from build123d import *

# Parameters (mm, degrees)
F0_W      = 482.6
F0_H      = 482.6
F1_DEPTH  = 12.8524
F2_W      = 330.2
F2_H      = 12.8524
F2_W_2    = 76.2
F3_DEPTH  = 50.8
F4_W      = 330.2
F4_H      = 12.8524
F4_W_2    = 76.2
F5_DEPTH  = 50.8
F8_W      = 127
F8_H      = 74.6771698952
F8_H_2    = 75.1828301048
F9_W      = 127
F9_H      = 74.6771698952
F10_DEPTH = 25.4
F12_DEPTH = 50.8
F13_DEPTH = 50.8
F14_R     = 30.353
F15_DEPTH = 25.4


with BuildPart() as f1:
    # F0 (on Top) → F1 (new body)
    with BuildSketch(Plane.XY):
        with Locations((-241.3, -241.3)):
            Rectangle(F0_W, F0_H)
    extrude(amount=F1_DEPTH)

    # F2 (on face) → F3 (cut)
    with BuildSketch(Plane.XZ.offset(482.6)):
        with Locations((-241.3, 6.4262)):
            Rectangle(F2_W, F2_H)
        with Locations((-444.5, 6.4262)):
            Rectangle(F2_W_2, F2_H)
    extrude(amount=-F3_DEPTH, mode=Mode.SUBTRACT)

    # F4 (on face) → F5 (cut)
    with BuildSketch(Plane(origin=(0, 0, 0), x_dir=(-1, 0, 0), z_dir=(0, 1, 0))):
        with Locations((241.3, 6.4262)):
            Rectangle(F4_W, F4_H)
        with Locations((38.1, 6.4262)):
            Rectangle(F4_W_2, F4_H)
    extrude(amount=-F5_DEPTH, mode=Mode.SUBTRACT)

    # F8 (on face) + F9 (on face) → F10 (cut)
    with BuildSketch(Plane.XY.offset(12.8524)):
        with Locations((-139.7, -318.2614150524)):
            Rectangle(F8_W, F8_H)
        with Locations((-342.9, -164.5914150524)):
            Rectangle(F8_W, F8_H_2)
        with Locations((-139.7, -164.5914150524)):
            Rectangle(F8_W, F8_H_2)
    with BuildSketch(Plane.XY.offset(12.8524)):
        with Locations((-342.9, -318.2614150524)):
            Rectangle(F9_W, F9_H)
    extrude(amount=-F10_DEPTH, mode=Mode.SUBTRACT)

    # F12 (cut): a face of the model
    f12_faces = [f1.faces().sort_by_distance(p)[0] for p in [
        (-38.1, -482.6, 6.4262),
    ]]
    extrude(f12_faces, amount=-F12_DEPTH, mode=Mode.SUBTRACT)

    # F13 (cut): a face of the model
    f13_faces = [f1.faces().sort_by_distance(p)[0] for p in [
        (-444.5, 0, 6.4262),
    ]]
    extrude(f13_faces, amount=-F13_DEPTH, mode=Mode.SUBTRACT)

    # F14 (on face) → F15 (cut)
    with BuildSketch(Plane.XY.offset(12.8524)):
        with Locations((-241.3, -241.5528301048)):
            Circle(F14_R)
    extrude(amount=-F15_DEPTH, mode=Mode.SUBTRACT)


solid = f1.part
Source: CAD feature listing. Evaluate the final solid. Frame: model axes, mm. A direction names the side the tool comes from. Round coordinates to 2 decimals unless told otherwise and drop trailing zeros. Loops run counter-clockwise (first coordinate to the right, second up) from the corner with the lowest first, then second, coordinate; pieces in that order, holes last. Notation, with made-up numbers: M 32,-18.75 L 64,-18.75 A34 cw 64,19.25 Z; hole C -34.5,89 d7. An arc over 180 degrees is marked long. Answer as CSV lines item,"result".
Q1. Pull-direction query (X, two-part tool) for faces 3 (the face through (-245, -196, 0)), 4 (the face through (-76.2, -165, 7)), 5 (the face through (-76.2, -319, 7)), 6 (the face through (0, -244, 6)); classes: +X half, -X half, draft (parallel to the pull), parting line (faces both ways), or undercut.
Verdict:
face 3,"draft"
face 4,"undercut"
face 5,"undercut"
face 6,"+X half"
Q2. Cut plane C-C (x = -241.3). Return the cut outline in (y, z), plus the area to 3 significant figures.
Verdict:
outline,"M -431.8,0 L -271.91,0 L -271.91,12.85 L -431.8,12.85 Z; M -211.2,0 L -50.8,0 L -50.8,12.85 L -211.2,12.85 Z"
area,"4,120 mm^2"
Q3. Cut plane B-B (y = -191.5). Return the cut outline in (x, z), plus the area to 3 significant figures.
Verdict:
outline,"M -482.6,0 L -406.4,0 L -406.4,12.85 L -482.6,12.85 Z; M -279.4,0 L -203.2,0 L -203.2,12.85 L -279.4,12.85 Z; M -76.2,0 L 0,0 L 0,12.85 L -76.2,12.85 Z"
area,"2,940 mm^2"
Q4. Contact query for a flat-ended pin moving along its axis: pin 1 (4 mm diameter, centred on y = -173, z = 5, fed in from +X). Output: stop coordinate, or through.
Verdict:
pin 1,"stops at x = 0"
Q5. Cut plane A-A (x = -377). Return the cut outline in (y, z).
Verdict:
outline,"M -431.8,0 L -355.6,0 L -355.6,12.85 L -431.8,12.85 Z; M -280.92,0 L -202.18,0 L -202.18,12.85 L -280.92,12.85 Z; M -127,0 L -50.8,0 L -50.8,12.85 L -127,12.85 Z"
Q6. Cut plane D-D (z = 9.25). Return the cut outline in (x, y), plus the area to 3 significant figures.
Verdict:
outline,"M -482.6,-431.8 L 0,-431.8 L 0,-50.8 L -482.6,-50.8 Z; hole M -406.4,-355.6 L -279.4,-355.6 L -279.4,-280.92 L -406.4,-280.92 Z; hole M -406.4,-202.18 L -279.4,-202.18 L -279.4,-127 L -406.4,-127 Z; hole C -241.3,-241.55 d60.71; hole M -203.2,-355.6 L -76.2,-355.6 L -76.2,-280.92 L -203.2,-280.92 Z; hole M -203.2,-202.18 L -76.2,-202.18 L -76.2,-127 L -203.2,-127 Z"
area,"143,000 mm^2"
Q7. Reachability of faces 1 (the face through (-245, -50.8, 6)), 2 (the face through (-344, -127, 7)) from +Z, -Z, +X, -X, +Y, -Y: full face, straight path, thin tool, end or side. Return the list, or none.
Verdict:
face 1,"+Z, -Z, +X, -X, +Y"
face 2,"+Z, -Z"
Q8. Line query: line 1 along Y through (x, z) = (-87, 11); line 2 along X through (y, z) = (-281, 8.25); line 3 along Y through (x, z) = (-241.3, 7.75). Output: solid intervals per line, ascending.
Verdict:
line 1,"y = -431.8 to -355.6, -280.92 to -202.18, -127 to -50.8"
line 2,"x = -482.6 to -406.4, -279.4 to -203.2, -76.2 to 0"
line 3,"y = -431.8 to -271.91, -211.2 to -50.8"
